Geometry check sheet. Reference: drawing and pictorial views, mm from the part's lowest x, y, z. A direction names the side the tool comes from. Give positions to 0.01 mm unless a question says otherwise; leave off trailing zeros. Write each loop counter-clockwise with the first axis right and the second up, starting at its lowest first coordinate (ties: lowest second). Pieces come first, ordered by that corner, then holes.
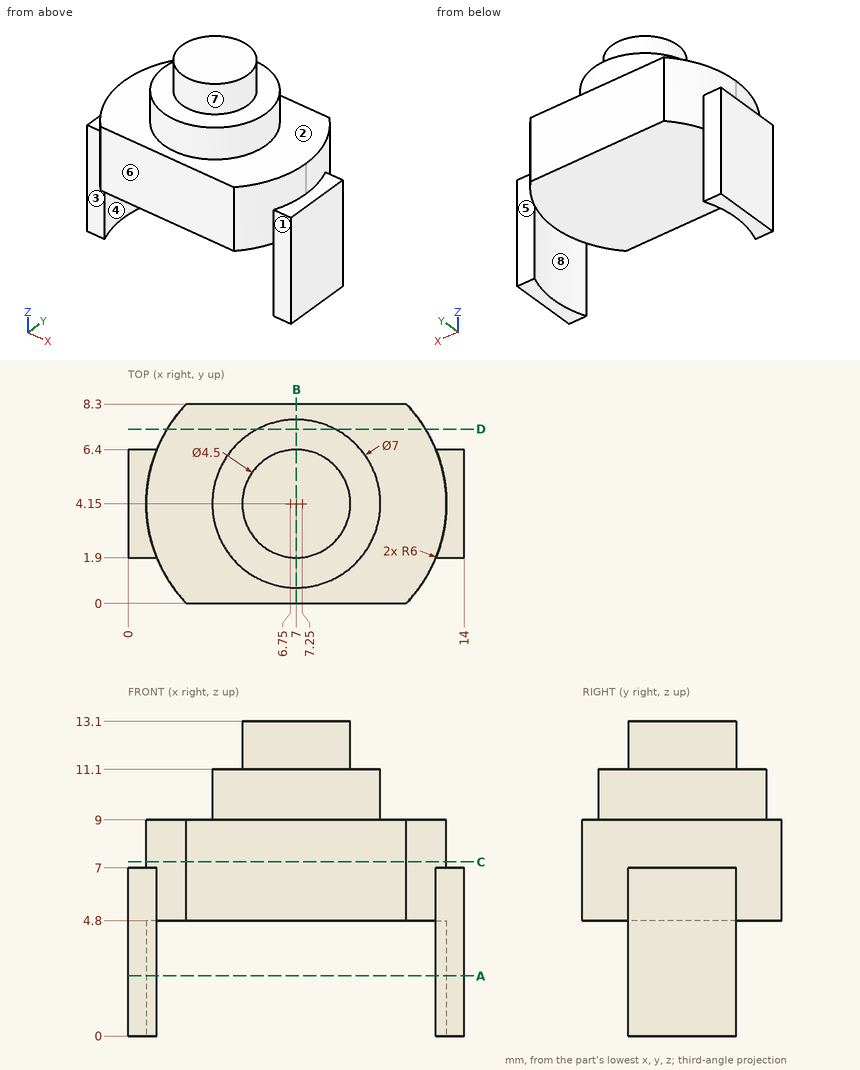
Item 1: Sectioned sample at C-C on z = 7.25. Record the cut outline in (x, y), then the cut area to 3 significant figures.
Answer key:
outline: (2.42, 0) - (11.58, 0) arc R6 ccw to (11.58, 8.3) - (2.42, 8.3) arc R6 ccw to start
area: 95.1 mm2
Item 2: Sectioned sample at D-D on y = 7.25. Record the cut outline in (x, z), then the cut area to 3 significant figures.
Answer key:
outline: (1.61, 4.8) - (12.39, 4.8) - (12.39, 9) - (8.62, 9) - (8.62, 11.1) - (5.38, 11.1) - (5.38, 9) - (1.61, 9) - close
area: 52.1 mm2
Item 3: Depth check by flat-ended pin: pin 1 (1.3 mm diameter, centred on x = 0.5, z = 5, fed in from -Y); pin 2 (4 mm diameter, centred on x = 9, y = 5, fed in from -Z); pin 3 (1 mm diameter, centred on y = 1, z = 6, fed in from +X); pin 4 (1 mm diameter, centred on y = 1, z = 4, fed in from -X). Enter the tip coordinate at first touch or a pass-through.
Answer key:
pin 1: stops at y = 1.9
pin 2: stops at z = 4.8
pin 3: stops at x = 12.63
pin 4: passes through
Item 4: Sectioned sample at A-A on z = 2.5. Record the cut outline in (x, y), then the cut area to 3 significant figures.
Answer key:
outline: (0, 1.9) - (1.19, 1.9) arc R6 cw to (1.19, 6.4) - (0, 6.4) - close; (12.81, 1.9) - (14, 1.9) - (14, 6.4) - (12.81, 6.4) arc R6 cw to start
area: 8.04 mm2
Item 5: Sectioned sample at B-B on x = 7. Record the cut outline in (y, z), then the cut area to 3 significant figures.
Answer key:
outline: (0, 4.8) - (8.3, 4.8) - (8.3, 9) - (7.65, 9) - (7.65, 11.1) - (6.4, 11.1) - (6.4, 13.1) - (1.9, 13.1) - (1.9, 11.1) - (0.65, 11.1) - (0.65, 9) - (0, 9) - close
area: 58.6 mm2
Item 6: Scan lines: line 1 along Z through (x, y) = (8, 4.5); line 2 along X through (y, z) = (4, 10.75); line 3 along Z through (x, y) = (1.25, 6). Record each from-to range of solid material in increasing order.
Answer key:
line 1: z = 4.8 to 13.1
line 2: x = 3.5 to 10.5
line 3: z = 4.8 to 9
Item 7: Release check for a two-part mould opening along Y. For the marked faces 6, 7 and 8 record: released by +Y, released by -Y, zero draft, split by the parting line, or undercut.
Answer key:
face 6: released by -Y
face 7: split by the parting line
face 8: undercut
Item 8: Set-up check for the marked faces 1, 2, 3, 4 and 5: record each of +Z, -Z, +X, -X, +Y, -Y from which the full face is reachable in a straight line by a thin tool's end or side.
Answer key:
face 1: +Z, -Z, +X, -Y
face 2: +Z
face 3: +Z, -Z, -X, -Y
face 4: -Z
face 5: +Z, -Z, +X, +Y
